from build123d import *

# Parameters (mm, degrees)
SKETCH_1_W           = 48
SKETCH_1_H           = 31
SKETCH_1_R           = 8.9
EXTRUDE_1_DEPTH      = 65
SKETCH_2_R           = 10.5
CUT_EXTRUDE_1_DEPTH  = 49
CUT_EXTRUDE_3_DEPTH  = 76.907838857
EXTRUDE_4_DEPTH      = 8
SKETCH_11_R          = 1.25
CUT_EXTRUDE_9_DEPTH  = 80.511005658
SKETCH_15_W          = 40.1
SKETCH_15_H          = 9.5
CUT_EXTRUDE_11_DEPTH = 80.511005658
SKETCH_17_R          = 1.6
CUT_EXTRUDE_13_DEPTH = 85.150163426
SKETCH_19_W          = 3
SKETCH_19_H          = 3
CUT_EXTRUDE_14_DEPTH = 76.651107105
EXTRUDE_5_DEPTH      = 8
EXTRUDE_START        = 1
EXTRUDE_6_DEPTH      = 1
CUT_EXTRUDE_START    = -10
SKETCH_22_R          = 1.25
CUT_EXTRUDE_15_DEPTH = 10
SKETCH_23_R          = 1.25
CUT_EXTRUDE_16_DEPTH = 7


with BuildPart() as part:
    # 草图1 → 凸台-拉伸1 (new body)
    with BuildSketch(Plane.XY):
        Rectangle(SKETCH_1_W, SKETCH_1_H)
        with Locations((0, -0.6)):
            Circle(SKETCH_1_R, mode=Mode.SUBTRACT)
    extrude(amount=EXTRUDE_1_DEPTH)

    # 草图2 → 切除-拉伸1 (cut)
    with BuildSketch(Plane.XY.offset(65)):
        with Locations((0, -0.6)):
            Circle(SKETCH_2_R)
    extrude(amount=-CUT_EXTRUDE_1_DEPTH, mode=Mode.SUBTRACT)

    # 草图4 → 切除-拉伸3 (cut, through all)
    with BuildSketch(Plane(origin=(0, 15.5, 0), x_dir=(1, 0, 0), z_dir=(0, 1, 0))):
        with BuildLine():
            Line((-24, 9), (-10.857864376, -4.142135624))
            ThreePointArc((-10.857864376, -4.142135624), (-6.52240935, -10.6306026), (-5, -18.284271247))
            Line((-5, -18.284271247), (-5, -29.715728753))
            ThreePointArc((-5, -29.715728753), (-6.52240935, -37.3693974), (-10.857864376, -43.857864376))
            ThreePointArc((-10.857864376, -43.857864376), (-16.798925034, -49.531146093), (-24, -53.484226727))
            Line((-24, -53.484226727), (-24, 9))
        make_face()
        with BuildLine():
            Line((5, -18.284271247), (5, -29.715728753))
            ThreePointArc((5, -29.715728753), (6.52240935, -37.3693974), (10.857864376, -43.857864376))
            ThreePointArc((10.857864376, -43.857864376), (16.798925034, -49.531146093), (24, -53.484226727))
            Line((24, -53.484226727), (24, 9))
            Line((24, 9), (10.857864376, -4.142135624))
            ThreePointArc((10.857864376, -4.142135624), (6.52240935, -10.6306026), (5, -18.284271247))
        make_face()
    extrude(amount=-CUT_EXTRUDE_3_DEPTH, mode=Mode.SUBTRACT)

    # 草图12 → 凸台-拉伸4 (add)
    with BuildSketch(Plane.XZ.offset(15.5)):
        with BuildLine():
            Line((-5, 18.284271247), (5, 18.284271247))
            Line((5, 18.284271247), (5, 29.715728753))
            ThreePointArc((5, 29.715728753), (6.52240935, 37.3693974), (10.857864376, 43.857864376))
            ThreePointArc((10.857864376, 43.857864376), (16.798925034, 49.531146093), (24, 53.484226727))
            Line((24, 53.484226727), (24, 65))
            Line((24, 65), (-24, 65))
            Line((-24, 65), (-24, 53.484226727))
            ThreePointArc((-24, 53.484226727), (-16.798925034, 49.531146093), (-10.857864376, 43.857864376))
            ThreePointArc((-10.857864376, 43.857864376), (-6.52240935, 37.3693974), (-5, 29.715728753))
            Line((-5, 29.715728753), (-5, 18.284271247))
        make_face()
    extrude(amount=EXTRUDE_4_DEPTH)

    # 草图11 → 切除-拉伸9 (cut, through all)
    with BuildSketch(Plane(origin=(0, 15.5, 0), x_dir=(1, 0, 0), z_dir=(0, 1, 0))):
        with Locations(Location((14, -51.5, 0), (0, 0, 270))):
            Circle(SKETCH_11_R)
        with Locations(Location((-14, -51.5, 0), (0, 0, 270))):
            Circle(SKETCH_11_R)
    extrude(amount=-CUT_EXTRUDE_9_DEPTH, mode=Mode.SUBTRACT)

    # 草图15 → 切除-拉伸11 (cut, through all)
    with BuildSketch(Plane(origin=(0, 15.5, 0), x_dir=(1, 0, 0), z_dir=(0, 1, 0))):
        with Locations((0, -60.25)):
            Rectangle(SKETCH_15_W, SKETCH_15_H)
    extrude(amount=-CUT_EXTRUDE_11_DEPTH, mode=Mode.SUBTRACT)

    # 草图17 → 切除-拉伸13 (cut, through all)
    with BuildSketch(Plane(origin=(24, 0, 0), x_dir=(0, 0, -1), z_dir=(1, 0, 0))):
        with Locations((-61.7, 9.8)):
            Circle(SKETCH_17_R)
        with Locations((-61.7, -3.8)):
            Circle(SKETCH_17_R)
        with BuildLine():
            Line((-55.5, -23.5), (-55.5, -6.8))
            Line((-55.5, -6.8), (-61.7, -6.8))
            ThreePointArc((-61.7, -6.8), (-63.821320344, -5.921320344), (-64.7, -3.8))
            Line((-64.7, -3.8), (-64.7, 9.8))
            ThreePointArc((-64.7, 9.8), (-63.821320344, 11.921320344), (-61.7, 12.8))
            Line((-61.7, 12.8), (-55.5, 12.8))
            Line((-55.5, 12.8), (-55.5, 15.5))
            Line((-55.5, 15.5), (-64.7, 15.5))
            Line((-64.7, 15.5), (-94.5, 15.5))
            Line((-94.5, 15.5), (-94.5, -23.5))
            Line((-94.5, -23.5), (-55.5, -23.5))
        make_face()
    extrude(amount=-CUT_EXTRUDE_13_DEPTH, mode=Mode.SUBTRACT)

    # 草图19 → 切除-拉伸14 (cut, through all)
    with BuildSketch(Plane.XZ.offset(15.5)):
        with Locations((-13.5, 1.5)):
            Rectangle(SKETCH_19_W, SKETCH_19_H)
        with Locations((13.5, 1.5)):
            Rectangle(SKETCH_19_W, SKETCH_19_H)
    extrude(amount=-CUT_EXTRUDE_14_DEPTH, mode=Mode.SUBTRACT)

    # 草图20 → 凸台-拉伸5 (add)
    with BuildSketch(Plane.XZ.offset(15.5)):
        with BuildLine():
            Line((-10.857864376, 4.142135624), (-12, 3))
            Line((-12, 3), (-12, 0))
            Line((-12, 0), (12, 0))
            Line((12, 0), (12, 3))
            Line((12, 3), (10.857864376, 4.142135624))
            ThreePointArc((10.857864376, 4.142135624), (6.52240935, 10.6306026), (5, 18.284271247))
            Line((5, 18.284271247), (-5, 18.284271247))
            ThreePointArc((-5, 18.284271247), (-6.52240935, 10.6306026), (-10.857864376, 4.142135624))
        make_face()
    extrude(amount=EXTRUDE_5_DEPTH)

    # 草图21 → 凸台-拉伸6 (add)
    with BuildSketch(Plane(origin=(0, 15.5, 0), x_dir=(1, 0, 0), z_dir=(0, 1, 0)).offset(EXTRUDE_START)):
        with BuildLine():
            Line((12, 0), (-12, 0))
            Line((-12, 0), (-12, -3))
            Line((-12, -3), (-10.857864376, -4.142135624))
            ThreePointArc((-10.857864376, -4.142135624), (-6.52240935, -10.6306026), (-5, -18.284271247))
            Line((-5, -18.284271247), (-5, -29.715728753))
            ThreePointArc((-5, -29.715728753), (-6.52240935, -37.3693974), (-10.857864376, -43.857864376))
            ThreePointArc((-10.857864376, -43.857864376), (-16.798925034, -49.531146093), (-24, -53.484226727))
            Line((-24, -53.484226727), (-24, -55.5))
            Line((-24, -55.5), (24, -55.5))
            Line((24, -55.5), (24, -53.484226727))
            ThreePointArc((24, -53.484226727), (16.798925034, -49.531146093), (10.857864376, -43.857864376))
            ThreePointArc((10.857864376, -43.857864376), (6.52240935, -37.3693974), (5, -29.715728753))
            Line((5, -29.715728753), (5, -18.284271247))
            ThreePointArc((5, -18.284271247), (6.52240935, -10.6306026), (10.857864376, -4.142135624))
            Line((10.857864376, -4.142135624), (12, -3))
            Line((12, -3), (12, 0))
        make_face()
    extrude(amount=-EXTRUDE_6_DEPTH)

    # 草图22 → 切除-拉伸15 (cut)
    with BuildSketch(Plane.XZ.offset(-15.5).offset(CUT_EXTRUDE_START)):
        with Locations(Location((-14, 51.5, 0), (0, 0, 90))):
            Circle(SKETCH_22_R)
        with Locations(Location((14, 51.5, 0), (0, 0, 90))):
            Circle(SKETCH_22_R)
    extrude(amount=CUT_EXTRUDE_15_DEPTH, mode=Mode.SUBTRACT)

    # 草图23 → 切除-拉伸16 (cut)
    with BuildSketch(Plane.XZ.offset(23.5)):
        with Locations(Location((0, 6, 0), (0, 0, 270))):
            Circle(SKETCH_23_R)
    extrude(amount=-CUT_EXTRUDE_16_DEPTH, mode=Mode.SUBTRACT)


solid = part.part
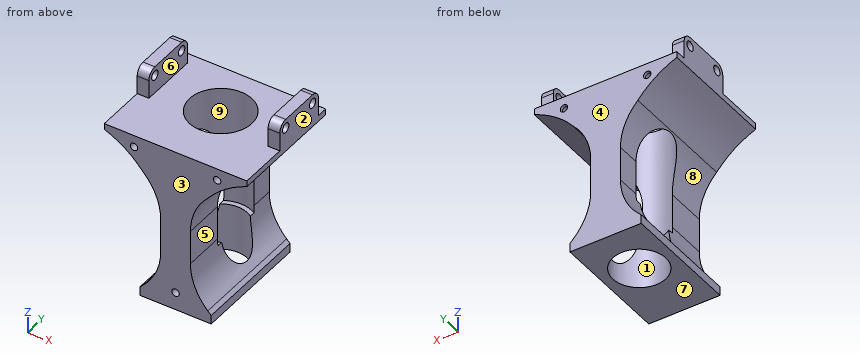
Source: CAD feature listing. Evaluate the final solid. Frame: model axes, mm. Face numbers are marked on the shaded views. A direction names the side the tool comes from. Coordinates: 2 decimals unless noted, no trailing zeros. Order: outer loops, then holes, each group sorted by start corner. A loop starts at its lowest first (then second) coordinate and runs counter-clockwise, first axis right, second up. Notation, with made-up numbers: M -9.5,-37.5 L 39.5,-37.5 A23 cw 39.5,-19.5 Z; hole C 77.25,23.25 d3. An arc over 180 degrees is marked long. Write each question's results on one line, items separated by ' | '. Start each with the question number.
1. Material intervals for L1, parallel to Y at x = -20.95, z = 61.7; L2, parallel to Y at x = 0, z = 36.5; L3, parallel to Z at x = 3, y = -18.5, sorted ascending.
2. Section B-B, the plane x = 0. Return the cut outline in (y, z).
3. Section D-D, the plane z = 51.5. Return the cut outline in (x, y).
4. Section A-A, the plane z = 28.5. Return the cut outline in (x, y).
5. Reachability of the marked faces 5, 6, 7, 8 and 9 from +Z, -Z, +X, -X, +Y, -Y: full face, straight path, thin tool, end or side. Return the list, or none.
6. Pin query (flat end, axial travel): pin 1 (0.8 mm diameter, centred on x = 0.5, z = 6, fed in from -Y); pin 2 (12 mm diameter, centred on x = -10, y = -12, fed in from +Z); pin 3 (1.6 mm diameter, centred on x = 1, y = -10, fed in from +Z). Return the tip coordinate at first contact, or that it passes through.
7. Draft query along Y for the marked faces 1, 2, 3 and 4. Return one class per face: +Y half, -Y half, draft (parallel to the pull), parting line (faces both ways), or undercut.
8. Section C-C, the plane y = -12. Return the cut outline in (x, z).
Solution:
1) L1: -6.8 to -5.4, -2.2 to 8.2, 11.4 to 12.8 | L2: -23.5 to -11.1, 9.9 to 16.5 | L3: 0 to 55.5
2) outline: M -23.5,0 L -9.5,0 L -9.5,16 L -11.1,16 L -11.1,55.5 L -23.5,55.5 L -23.5,7.25 L -16.5,7.25 L -16.5,4.75 L -23.5,4.75 Z; M 8.3,0 L 16.5,0 L 16.5,55.5 L 9.9,55.5 L 9.9,16 L 8.3,16 Z
3) outline: M -19.84,-23.5 L -15.25,-23.5 L -15.25,16.5 L -19.84,16.5 Z; M -12.75,-23.5 L 12.75,-23.5 L 12.75,16.5 L -12.75,16.5 Z; M 15.25,-23.5 L 19.84,-23.5 L 19.84,16.5 L 15.25,16.5 Z; hole C 0,-0.6 d21
4) outline: M -5,-23.5 L 5,-23.5 L 5,-9.83 A10.5 cw -5,-9.83 Z; M -5,8.63 A10.5 cw 5,8.63 L 5,16.5 L -5,16.5 Z
5) face 5: +X, +Y, -Y | face 6: +Z, +Y, -Y | face 7: -Z, +X, -X, +Y, -Y | face 8: -X, +Y, -Y | face 9: +Z
6) pin 1: y = -16.5 | pin 2: z = 55.5 | pin 3: z = 16
7) face 1: undercut | face 2: draft | face 3: -Y half | face 4: +Y half
8) outline: M -24,53.48 A31.65 cw -10.86,43.86 A20 cw -5,29.72 L -5,18.28 A20 cw -10.86,4.14 L -12,3 L -12,0 L 12,0 L 12,3 L 10.86,4.14 A20 cw 5,18.28 L 5,29.72 A20 cw 10.86,43.86 A31.65 cw 24,53.48 L 24,55.5 L -24,55.5 Z; hole C -14,51.5 d2.5; hole C 14,51.5 d2.5
